Geometry: final body of the model. Coordinates: model frame, mm. A direction names the side the tool comes from. Coordinates: 2 decimals unless noted, no trailing zeros. Order: outer loops, then holes, each group sorted by start corner. A loop starts at its lowest first (then second) coordinate and runs counter-clockwise, first axis right, second up. Notation, with made-up numbers: (79.25, 6) - (133.25, 6) arc R27 cw to (133.25, 37) - close; hole circle Ø10 at (21, 42). An arc over 180 degrees is marked (long way). Use one line per item in the form item = value. Start each with the question number.
```python
from build123d import *

# Parameters (mm, degrees)
ESQUISSE1_R        = 10
BOSS_EXTRU_1_DEPTH = 10


with BuildPart() as part:
    # Esquisse1 → Boss.-Extru.1 (new body)
    # profile 1 of 3: a face of its own
    with BuildSketch(Plane.XY):
        with BuildLine():
            Line((36.568542495, 156.568542495), (36.568542495, 64.852813742))
            Line((36.568542495, 64.852813742), (42.426406871, 70.710678119))
            ThreePointArc((42.426406871, 70.710678119), (64.222211142, 75.046133145), (76.568542495, 56.568542495))
            Line((76.568542495, 56.568542495), (76.568542495, 156.568542495))
            ThreePointArc((76.568542495, 156.568542495), (56.568542495, 176.568542495), (36.568542495, 156.568542495))
        make_face()
        with Locations((56.568542495, 156.568542495)):
            Circle(ESQUISSE1_R, mode=Mode.SUBTRACT)
    # profile 2 of 3: a face of its own
    with BuildSketch(Plane.XY):
        with BuildLine():
            Line((42.426406871, 70.710678119), (36.568542495, 64.852813742))
            Line((36.568542495, 64.852813742), (36.568542495, 56.568542495))
            ThreePointArc((36.568542495, 56.568542495), (48.914873848, 38.090951845), (70.710678119, 42.426406871))
            ThreePointArc((70.710678119, 42.426406871), (75.046133145, 48.914873848), (76.568542495, 56.568542495))
            ThreePointArc((76.568542495, 56.568542495), (64.222211142, 75.046133145), (42.426406871, 70.710678119))
        make_face()
    # profile 3 of 3: a face of its own
    with BuildSketch(Plane.XY):
        with BuildLine():
            Line((36.568542495, 64.852813742), (-14.142135624, 14.142135624))
            ThreePointArc((-14.142135624, 14.142135624), (-14.142135624, -14.142135624), (14.142135624, -14.142135624))
            Line((14.142135624, -14.142135624), (70.710678119, 42.426406871))
            ThreePointArc((70.710678119, 42.426406871), (48.914873848, 38.090951845), (36.568542495, 56.568542495))
            Line((36.568542495, 56.568542495), (36.568542495, 64.852813742))
        make_face()
        Circle(ESQUISSE1_R, mode=Mode.SUBTRACT)
    extrude(amount=BOSS_EXTRU_1_DEPTH)


solid = part.part
```
(1) Cut plane C-C on y = 6. Return the cut outline in (x, z).
(2) Cut plane D-D on y = 69.5. Return the cut outline in (x, z).
(3) Cut plane A-A on x = 3. Return the cut outline in (y, z).
(4) Draft query along X for faces 1 (the flat face through (49, 80, 0)), 2 (the cylindrical face through (75, 48.8, 4.9)), 3 (the cylindrical face through (54.401, 146.806, 4.93)), 4 (the cylindrical face through (57.008, 176.564, 4.93)). Return one class per face: released by +X, released by -X, zero draft, split by the parting line, or undercut.
(5) Contact query for flat-ended pins moving along their axis: pin 1 Ø1.5 at (x, z) = (30.5, 4.5) entering from +Y; pin 2 Ø5 at (x, z) = (35.5, 2.5) entering from -Y; pin 3 Ø5 at (y, z) = (46.5, 8) entering from +X. Output: stop coordinate, or through.
(6) Material intervals for L1, parallel to Y at x = 0, z = 6.75; L2, parallel to X at y = 123, z = 8; L3, parallel to Y at x = 7, z = 0.5 (3 decimals), sorted ascending. Write a range as from..to.
(7) Set-up query: faces 5 (the flat face through (36.569, 111, 5)), 6 (the flat face through (49, 80, 10)). Return all of +Z, -Z, +X, -X, +Y, -Y with unobstructed straight access to the full face (end or side cutting, diameter ignored); none if empty.
(8) Cut plane B-B on z = 7. Return the cut outline in (x, y).
Check sheet entries:
q1.outline = (-19.08, 0) - (-8, 0) - (-8, 10) - (-19.08, 10) - close; (8, 0) - (34.28, 0) - (34.28, 10) - (8, 10) - close
q2.outline = (36.57, 0) - (76.57, 0) - (76.57, 10) - (36.57, 10) - close
q3.outline = (-19.77, 0) - (-9.54, 0) - (-9.54, 10) - (-19.77, 10) - close; (9.54, 0) - (31.28, 0) - (31.28, 10) - (9.54, 10) - close
q4.face_1 = zero draft
q4.face_2 = released by +X
q4.face_3 = undercut
q4.face_4 = split by the parting line
q5.pin_1 = 59.53
q5.pin_2 = 4.72
q5.pin_3 = 75.08
q6.L1 = -20..-10, 10..28.28
q6.L2 = 36.57..76.57
q6.L3 = -18.735..-7.141, 7.141..35.284
q7.face_5 = +Z, -Z, -X, +Y
q7.face_6 = +Z, +X, -X, +Y, -Y
q8.outline = (-14.14, 14.14) arc R20 ccw to (14.14, -14.14) - (70.71, 42.43) arc R20 ccw to (76.57, 56.57) - (76.57, 156.57) arc R20 ccw to (36.57, 156.57) - (36.57, 64.85) - close; hole circle Ø20 at (0, 0); hole circle Ø20 at (56.57, 156.57)
